from build123d import *

# Parameters (mm, degrees)
F0_R     = 0.75
F1_DEPTH = 1
F2_DEPTH = 4.8
F4_DEPTH = 2


with BuildPart() as f1:
    # F0 (on Front) → F1 (new body, symmetric)
    with BuildSketch(Plane.XZ):
        with BuildLine():
            Line((-4, 0), (0, 0))
            Line((0, 0), (24, 0))
            ThreePointArc((24, 0), (25.75, 1.75), (24, 3.5))
            Line((24, 3.5), (0, 3.5))
            Line((0, 3.5), (-2.5, 4))
            Line((-2.5, 4), (-4, 4))
            ThreePointArc((-4, 4), (-2.585786, 3.414214), (-2, 2))
            ThreePointArc((-2, 2), (-2.585786, 0.585786), (-4, 0))
        make_face()
        with Locations((24, 1.75)):
            Circle(F0_R, mode=Mode.SUBTRACT)
        with BuildLine():
            ThreePointArc((-4, 4), (-6, 2), (-4, 0))
            ThreePointArc((-4, 0), (-2.585786, 0.585786), (-2, 2))
            ThreePointArc((-2, 2), (-2.585786, 3.414214), (-4, 4))
        make_face()
        with Locations((-4, 2)):
            Circle(F0_R, mode=Mode.SUBTRACT)
    extrude(amount=F1_DEPTH, both=True)

    # F0 (on Front) → F2 (join, symmetric)
    with BuildSketch(Plane.XZ):
        with BuildLine():
            ThreePointArc((-4, 4), (-6, 2), (-4, 0))
            ThreePointArc((-4, 0), (-2.585786, 0.585786), (-2, 2))
            ThreePointArc((-2, 2), (-2.585786, 3.414214), (-4, 4))
        make_face()
        with Locations((-4, 2)):
            Circle(F0_R, mode=Mode.SUBTRACT)
    extrude(amount=F2_DEPTH, both=True)

    # F3 (on Front) → F4 (join, symmetric)
    with BuildSketch(Plane.XZ):
        with BuildLine():
            Line((20.5, 3.5), (0, 3.5))
            Line((0, 3.5), (-3.022093, 3.5))
            Line((-3.022093, 3.5), (-3.022093, 2.5))
            Line((-3.022093, 2.5), (0, 2.5))
            Line((0, 2.5), (20.5, 2.5))
            ThreePointArc((20.5, 2.5), (21.25, 1.75), (20.5, 1))
            Line((20.5, 1), (-4, 1))
            Line((-4, 1), (-4, 0))
            Line((-4, 0), (20.5, 0))
            ThreePointArc((20.5, 0), (22.25, 1.75), (20.5, 3.5))
        make_face()
    extrude(amount=F4_DEPTH, both=True)


solid = f1.part
Check sheet for the modelled part. Datum: model origin and axes. Units: mm. A direction names the side the tool comes from. Coordinates: 2 decimals unless noted, no trailing zeros. Loops run counter-clockwise (first coordinate to the right, second up) from the corner with the lowest first, then second, coordinate; pieces in that order, holes last. Notation, with made-up numbers: (43.25, -26) -> (78.25, -26) arc R20 cw to (78.25, -2) -> close; hole circle Ø2 at (59, 15). An arc over 180 degrees is marked (long way). Answer in a Markdown table with one row per item.
1. Go/stop test with flat-tipped pins: pin 1 (1.5 mm diameter, centred on x = 10, z = 3.5, fed in from -Y); pin 2 (1 mm diameter, centred on y = -2, z = 1, fed in from -X); pin 3 (2 mm diameter, centred on x = 14, y = -1, fed in from +Z). Record where each tip stops, or that it passes through.
Check values:
| item | result |
|---|---|
| pin 1 | stops at y = -2 |
| pin 2 | stops at x = -5.94 |
| pin 3 | stops at z = 3.5 |
2. Access from +Z, -Z, +X, -X, +Y, -Y to the whole of each face (thin tool, end or side, straight path). Record for faces 1 (the face through (9, 1, 2)), 2 (the face through (-3, -4.8, 2)), 3 (the face through (9, -1, 2)), 4 (the face through (22.25, 1.49, 1.71)).
Check values:
| item | result |
|---|---|
| face 1 | +Y |
| face 2 | +Z, -Z, +X, -X, -Y |
| face 3 | -Y |
| face 4 | +X, +Y |
3. Release check for a two-part mould opening along X. For faces 5 (the face through (25.75, -0.01, 1.71)), 6 (the face through (23, 1, 2)), 7 (the face through (-4.75, 0.07, 2.03)) record: released by +X, released by -X, zero draft, split by the parting line, or undercut.
Check values:
| item | result |
|---|---|
| face 5 | released by +X |
| face 6 | zero draft |
| face 7 | undercut |
4. Sectioned sample at A-A, the plane x = 10.5. Record the boundary of the cut face in (y, z), then the cut area to 3 significant figures.
Check values:
| item | result |
|---|---|
| outline | (-2, 0) -> (2, 0) -> (2, 1) -> (1, 1) -> (1, 2.5) -> (2, 2.5) -> (2, 3.5) -> (-2, 3.5) -> (-2, 2.5) -> (-1, 2.5) -> (-1, 1) -> (-2, 1) -> close |
| area | 11.0 mm2 |
5. Sectioned sample at C-C, the plane z = 0.55. Record the boundary of the cut face in (x, y).
Check values:
| item | result |
|---|---|
| outline | (-5.38, -4.8) -> (-2.62, -4.8) -> (-2.62, -2) -> (21.77, -2) -> (21.77, -1) -> (25.27, -1) -> (25.27, 1) -> (21.77, 1) -> (21.77, 2) -> (-2.62, 2) -> (-2.62, 4.8) -> (-5.38, 4.8) -> close |
6. Sectioned sample at B-B, the plane y = 3.25. Record the boundary of the cut face in (x, z).
Check values:
| item | result |
|---|---|
| outline | (-4, 0) arc R2 ccw to (-2, 2) arc R2 ccw to (-4, 4) arc R2 ccw to start; hole circle Ø1.5 at (-4, 2) |
7. Material ranges on line 1 along Z through (x, y) = (-4, -2.5); line 2 along Z through (x, y) = (24, 0.4); line 3 along Y through (x, z) = (10, 3.35), recorded low to high. Write a range as [from, to].
Check values:
| item | result |
|---|---|
| line 1 | z = [0, 1.25], [2.75, 4] |
| line 2 | z = [0, 1], [2.5, 3.5] |
| line 3 | y = [-2, 2] |
